Here's the drawing with two shaded views (mm, measured from the low corner). I have some questions. A direction names the side the tool comes from. Round coordinates to 2 decimals unless told otherwise and drop trailing zeros. Order: outer loops, then holes, each group sorted by start corner. A loop starts at its lowest first (then second) coordinate and runs counter-clockwise, first axis right, second up. Notation, with made-up numbers: (20, -33) - (57, -33) arc R32 ccw to (57, -7) - close; hole circle Ø10 at (61, 44). An arc over 180 degrees is marked (long way). Return JSON: item names as keys, results as strings. Group by question number.
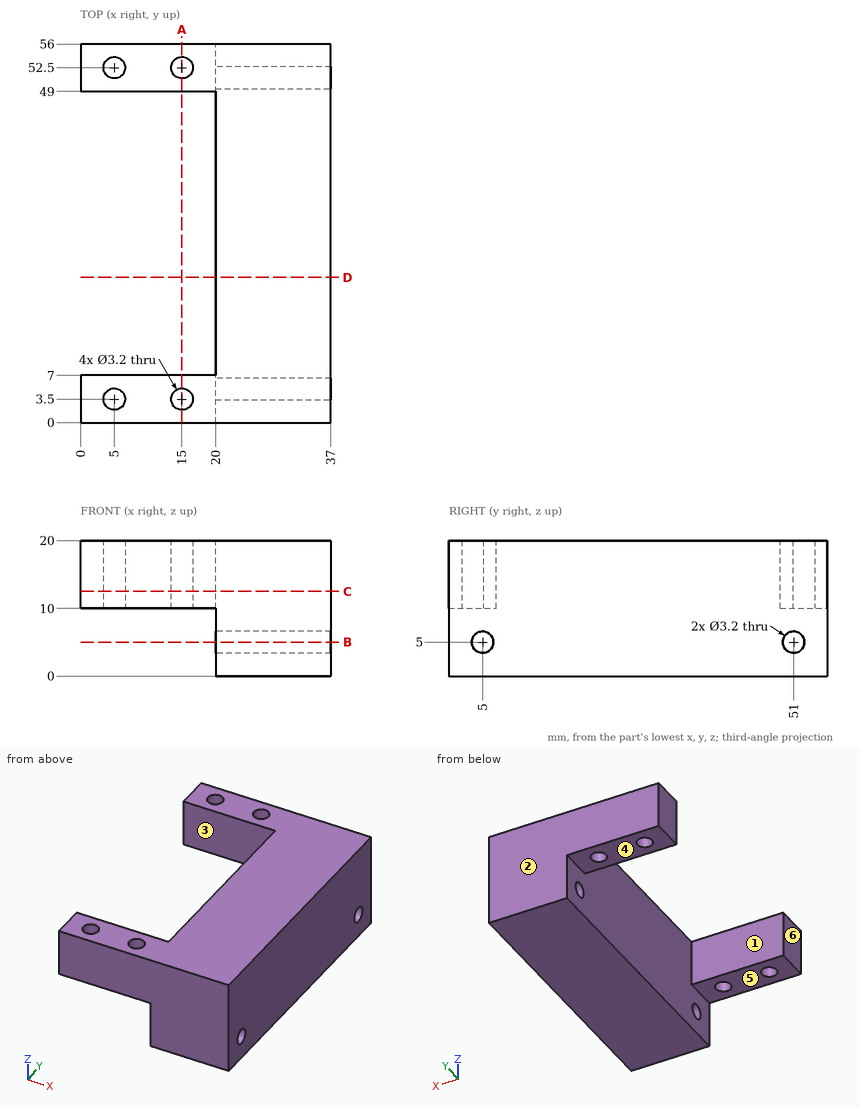
1) I want a section at C-C, the plane z = 12.5. List the corners of the cut face in (x, y) for me, plus the area to 3 significant figures.
2) I want a section at A-A, the plane x = 15. List the corners of the cut face in (y, z) for me.
3) We'd pull the mould along Y, two halves only. Please class the marked faces 1, 2, 3 and 4: +Y half, -Y half, draft (parallel to the pull), parting line (faces both ways), or undercut.
4) Will these pins go through, and if not, where does the flat tip stop? pin 1 (3 mm diameter, centred on x = 24.5, y = 20.5, fed in from -Z); pin 2 (4 mm diameter, centred on x = 15, y = 52.5, fed in from -Z); pin 3 (6 mm diameter, centred on y = 28.5, z = 8.5, fed in from -X).
5) I want a section at B-B, the plane z = 5. List the corners of the cut face in (x, y) for me.
6) If I drill on line 1 along Y through (x, z) = (5, 18); line 2 along Y through (x, z) = (33.5, 5); line 3 along Z through (x, y) = (30, 5), over which ranges is the centre line in solid material (lowest first)? Write a range as from..to.
7) I want a section at D-D, the plane y = 21.5. List the corners of the cut face in (x, z) for me.
8) For the marked faces 5 and 6, which set-ups out of +Z, -Z, +X, -X, +Y, -Y let a thin tool reach every point of the face, with its end or its side?
Outcome:
{
 "1": {"outline": "(0, 0) - (37, 0) - (37, 56) - (0, 56) - (0, 49) - (20, 49) - (20, 7) - (0, 7) - close; hole circle Ø3.2 at (5, 3.5); hole circle Ø3.2 at (5, 52.5); hole circle Ø3.2 at (15, 3.5); hole circle Ø3.2 at (15, 52.5)", "area": "1,200 mm^2"},
 "2": {"outline": "(0, 10) - (1.9, 10) - (1.9, 20) - (0, 20) - close; (5.1, 10) - (7, 10) - (7, 20) - (5.1, 20) - close; (49, 10) - (50.9, 10) - (50.9, 20) - (49, 20) - close; (54.1, 10) - (56, 10) - (56, 20) - (54.1, 20) - close"},
 "3": {"face 1": "undercut", "face 2": "+Y half", "face 3": "undercut", "face 4": "draft"},
 "4": {"pin 1": "z = 0", "pin 2": "z = 10", "pin 3": "x = 20"},
 "5": {"outline": "(20, 0) - (37, 0) - (37, 3.4) - (20, 3.4) - close; (20, 6.6) - (37, 6.6) - (37, 49.4) - (20, 49.4) - close; (20, 52.6) - (37, 52.6) - (37, 56) - (20, 56) - close"},
 "6": {"line 1": "0..1.9, 5.1..7, 49..50.9, 54.1..56", "line 2": "0..3.4, 6.6..49.4, 52.6..56", "line 3": "0..3.4, 6.6..20"},
 "7": {"outline": "(20, 0) - (37, 0) - (37, 20) - (20, 20) - close"},
 "8": {"face 5": "-Z, -X, +Y, -Y", "face 6": "+Z, -Z, -X, +Y, -Y"}
}
